Read the model definition and answer for the solid it produces. Units are mm, in the model's axes. Face numbers are marked on the shaded views. A direction names the side the tool comes from. Round coordinates to 2 decimals unless told otherwise and drop trailing zeros. Loops run counter-clockwise (first coordinate to the right, second up) from the corner with the lowest first, then second, coordinate; pieces in that order, holes last. Notation, with made-up numbers: M 71,13 L 80,13 A11 cw 80,32 Z; hole C -25,-20.5 d6. An arc over 180 degrees is marked long. Answer as CSV lines item,"result".
```python
from build123d import *

# Parameters (mm, degrees)
F0_W     = 20.32
F0_H     = 18.4829973394
F0_H_2   = 19.5233401282
F0_W_2   = 20.3507310414
F1_DEPTH = 25.4


with BuildPart() as f1:
    # F0 (on Front) → F1 (new body)
    with BuildSketch(Plane.XZ):
        with Locations((0, 6.7764989921)):
            Rectangle(F0_W, F0_H)
        with Locations((0, 25.7796677259)):
            Rectangle(F0_W, F0_H_2)
        with Locations((20.3353655207, 6.7764989921)):
            Rectangle(F0_W_2, F0_H)
        Polygon((-10.16, -2.4649996776), (-10.16, 16.0179976618), (-30.6711569428, 16.0179976618), (-30.6711569428, -2.8106316458), (-10.16, -2.8106316458), align=None)
    extrude(amount=F1_DEPTH)


solid = f1.part
```
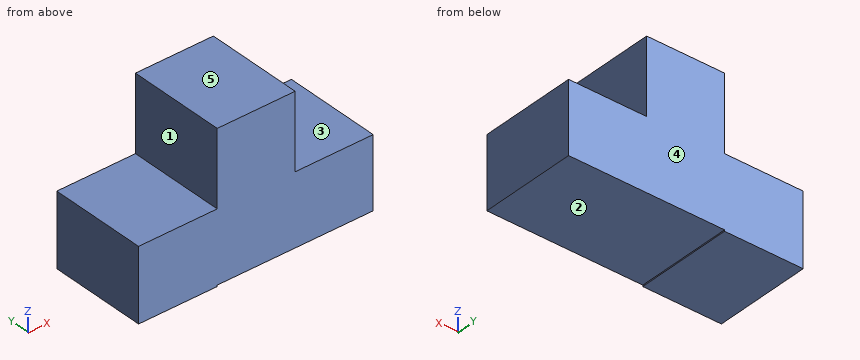
1) Find section C-C, the plane x = -12. Give the vertices of the cut face in (y, z), then the cut area to 3 significant figures.
Evaluation:
outline,"M -25.4,-2.81 L 0,-2.81 L 0,16.02 L -25.4,16.02 Z"
area,"478 mm^2"
2) Straight lines are drawn through the part: line 1 (Z direction, x = -10, y = -20.25) (3 decimals); line 2 (Z direction, x = 17, y = -17.25) (3 decimals); line 3 (X direction, y = -1.5, z = 25). For each, find the intervals that lie inside material, in ascending order.
Evaluation:
line 1,"z = -2.465 to 35.541"
line 2,"z = -2.465 to 16.018"
line 3,"x = -10.16 to 10.16"
3) Each of these flat-tipped pins is pushed along its axis until it touches: P1, Ø10, axis at y = -9.5, z = 24, coming from the -X side; P2, Ø6, axis at x = 25, y = -11.5, coming from the +Z side. Where does it stop, or does it pass through?
Evaluation:
P1,"stops at x = -10.16"
P2,"stops at z = 16.02"
4) Find section A-A, the plane y = -13.5. Give the vertices of the cut face in (x, z) (3 decimals).
Evaluation:
outline,"M -30.671,-2.811 L -10.16,-2.811 L -10.16,-2.465 L 30.511,-2.465 L 30.511,16.018 L 10.16,16.018 L 10.16,35.541 L -10.16,35.541 L -10.16,16.018 L -30.671,16.018 Z"
5) A tool of negligible diameter and unlimited length cuts with its end or side. For the marked faces 1, 2, 3, 4 and 5, from which of +Z, -Z, +X, -X, +Y, -Y can it reach the whole face along a straight path? Write none if from no direction.
Evaluation:
face 1,"+Z, -X, +Y, -Y"
face 2,"-Z, +X, +Y, -Y"
face 3,"+Z, +X, +Y, -Y"
face 4,"+Z, -Z, +X, -X, +Y"
face 5,"+Z, +X, -X, +Y, -Y"
6) Find section B-B, the plane z = 25.5. Give the vertices of the cut face in (x, y), then the cut area to 3 significant figures.
Evaluation:
outline,"M -10.16,-25.4 L 10.16,-25.4 L 10.16,0 L -10.16,0 Z"
area,"516 mm^2"
